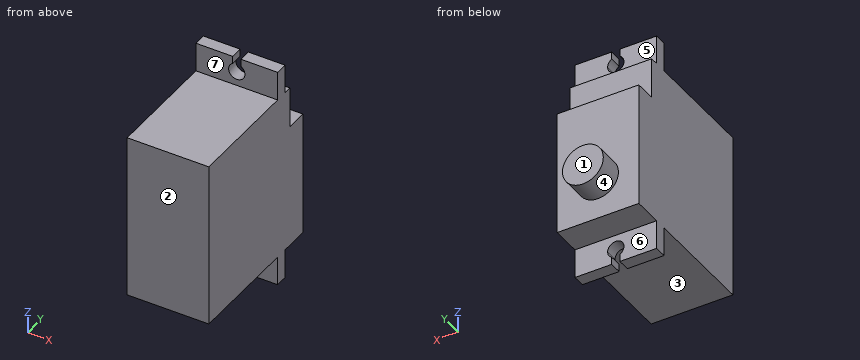
from build123d import *

# Parameters (mm, degrees)
SKETCH2_W           = 40.7
SKETCH2_H           = 32.8
SKETCH2_W_2         = 7.15
SKETCH2_H_2         = 3
BOSS_EXTRUDE1_DEPTH = 10
SKETCH3_R           = 5
BOSS_EXTRUDE2_DEPTH = 6.1
CUT_EXTRUDE1_DEPTH  = 43.483996987


with BuildPart() as part:
    # Sketch2 → Boss-Extrude1 (new, symmetric)
    with BuildSketch(Plane(origin=(0, 0, 0), x_dir=(0, 0, -1), z_dir=(1, 0, 0))):
        Rectangle(SKETCH2_W, SKETCH2_H)
        with Locations((-23.925, 12.9)):
            Rectangle(SKETCH2_W_2, SKETCH2_H_2)
        with Locations((23.925, 12.9)):
            Rectangle(SKETCH2_W_2, SKETCH2_H_2)
        Polygon((-10.35, 16.4), (20.35, 16.4), (20.35, 21.6), (15.35, 21.6), (5.35, 21.6), (-10.35, 21.6), align=None)
    extrude(amount=BOSS_EXTRUDE1_DEPTH, both=True)

    # Sketch3 → Boss-Extrude2 (add)
    with BuildSketch(Plane(origin=(0, 21.6, 0), x_dir=(1, 0, 0), z_dir=(0, 1, 0))):
        with Locations(Location((0, 10.35, 0), (0, 0, 270))):
            Circle(SKETCH3_R)
    extrude(amount=BOSS_EXTRUDE2_DEPTH)

    # Sketch4 → Cut-Extrude1 (cut, through all)
    with BuildSketch(Plane(origin=(0, 14.4, 0), x_dir=(1, 0, 0), z_dir=(0, 1, 0))):
        with BuildLine():
            Line((-1, -25.657050808), (-1, -27.5))
            Line((-1, -27.5), (1, -27.5))
            Line((1, -27.5), (1, -25.657050808))
            ThreePointArc((1, -25.657050808), (0, -25.925), (-1, -25.657050808))
        make_face()
        with BuildLine():
            ThreePointArc((2, -23.925), (-1, -22.192949192), (-1, -25.657050808))
            Line((-1, -25.657050808), (1, -25.657050808))
            ThreePointArc((1, -25.657050808), (1.732050808, -24.925), (2, -23.925))
        make_face()
        with BuildLine():
            Line((1, -25.657050808), (-1, -25.657050808))
            ThreePointArc((-1, -25.657050808), (0, -25.925), (1, -25.657050808))
        make_face()
        with BuildLine():
            ThreePointArc((2, 23.925), (1.732050808, 24.925), (1, 25.657050808))
            Line((1, 25.657050808), (-1, 25.657050808))
            ThreePointArc((-1, 25.657050808), (-1, 22.192949192), (2, 23.925))
        make_face()
        with BuildLine():
            Line((-1, 25.657050808), (1, 25.657050808))
            ThreePointArc((1, 25.657050808), (0, 25.925), (-1, 25.657050808))
        make_face()
        with BuildLine():
            Line((1, 25.657050808), (1, 27.5))
            Line((1, 27.5), (-1, 27.5))
            Line((-1, 27.5), (-1, 25.657050808))
            ThreePointArc((-1, 25.657050808), (0, 25.925), (1, 25.657050808))
        make_face()
    extrude(amount=-CUT_EXTRUDE1_DEPTH, mode=Mode.SUBTRACT)


solid = part.part
The model under review builds one solid part; all positions refer to its coordinate system, in mm. Face numbers are marked on the shaded views. A direction names the side the tool comes from. Give positions to 0.01 mm unless a question says otherwise; leave off trailing zeros. Write each loop counter-clockwise with the first axis right and the second up, starting at its lowest first coordinate (ties: lowest second). Pieces come first, ordered by that corner, then holes. Notation, with made-up numbers: M 66,27 L 88,27 A12 ccw 88,44 Z; hole C 57.25,33.25 d11. An arc over 180 degrees is marked long. One line per question, with ' | ' between items. Start each with the question number.
Item 1: We need section A-A on z = -10.35. Write out the cut boundary in (x, y), plus the area to 3 significant figures.
Item 2: We need section D-D on x = 0. Write out the cut boundary in (y, z) (3 decimals), plus the area to 3 significant figures.
Item 3: We need section C-C on x = 7.75. Write out the cut boundary in (y, z).
Item 4: We need section B-B on y = 13. Write out the cut boundary in (x, z) (3 decimals), plus the area to 3 significant figures.
Item 5: For the marked faces 4, 5, 6 and 7, list the 3-axis set-ups (+Z, -Z, +X, -X, +Y, -Y) from which the entire face can be reached by the end or side of a thin tool; tool diameter is ignored.
Item 6: Draft analysis for pull direction Y (two halves, no side actions). For the marked faces 1, 2 and 3, state which applies: released by +Y, released by -Y, zero draft, split by the parting line, or undercut.
Item 7: Wall thickness on line 1 (Y direction, x = 2.5, z = -18); line 2 (Z direction, x = -2, y = 19); line 3 (Z direction, x = 0.25, y = 10): over which ranges is each line inside the solid? List them lowest first. Write a range as from..to.
Item 8: For pin 1 (0.6 mm diameter, centred on x = -3, y = 15.5, fed in from +Z); pin 2 (6 mm diameter, centred on x = -4, y = 18.5, fed in from -Z); pin 3 (3 mm diameter, centred on x = 0, z = -23.925, fed in from +Y); pin 4 (3.5 mm diameter, centred on x = 1, z = 23.5, fed in from -Y), all flat-tipped, find the tip position at first contact; note any pin that passes through.
Results found:
1) outline: M -10,-16.4 L 10,-16.4 L 10,21.6 L 5,21.6 L 5,27.7 L -5,27.7 L -5,21.6 L -10,21.6 Z | area: 821 mm2
2) outline: M -16.4,-20.35 L 11.4,-20.35 L 11.4,-21.925 L 14.4,-21.925 L 14.4,-20.35 L 21.6,-20.35 L 21.6,-15.35 L 27.7,-15.35 L 27.7,-5.35 L 21.6,-5.35 L 21.6,10.35 L 16.4,10.35 L 16.4,20.35 L 14.4,20.35 L 14.4,21.925 L 11.4,21.925 L 11.4,20.35 L -16.4,20.35 Z | area: 1,570 mm2
3) outline: M -16.4,-20.35 L 11.4,-20.35 L 11.4,-27.5 L 14.4,-27.5 L 14.4,-20.35 L 21.6,-20.35 L 21.6,10.35 L 16.4,10.35 L 16.4,20.35 L 14.4,20.35 L 14.4,27.5 L 11.4,27.5 L 11.4,20.35 L -16.4,20.35 Z
4) outline: M -10,-27.5 L -1,-27.5 L -1,-25.657 A2 cw long 1,-25.657 L 1,-27.5 L 10,-27.5 L 10,27.5 L 1,27.5 L 1,25.657 A2 cw long -1,25.657 L -1,27.5 L -10,27.5 Z | area: 1,070 mm2
5) face 4: +Y | face 5: +Z, +X, -X, +Y | face 6: -Z, +X, -X, +Y | face 7: +Z, +X, -X, -Y
6) face 1: released by +Y | face 2: released by -Y | face 3: zero draft
7) line 1: y = -16.4..21.6 | line 2: z = -20.35..10.35 | line 3: z = -20.35..20.35
8) pin 1: stops at z = 20.35 | pin 2: stops at z = -20.35 | pin 3: passes through | pin 4: stops at y = 11.4
